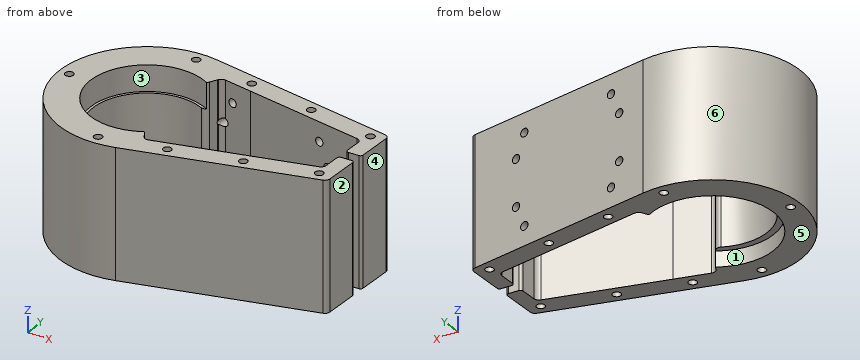
from build123d import *

# Parameters (mm, degrees)
EXTRUDE_1_DEPTH            = 50
SKETCH_2_R                 = 26
CUT_EXTRUDE_1_DEPTH        = 50
EXTRUDE_2_DEPTH            = 50
CUT_EXTRUDE_START          = -68
SKETCH_3_R                 = 1.6
CUT_EXTRUDE_2_DEPTH        = 68
CUT_EXTRUDE_1_2_DEPTH      = 143.467540163
CUT_EXTRUDE_1_2_DEPTH_BACK = 58
CUT_EXTRUDE_START_2        = -58
CUT_EXTRUDE_3_DEPTH        = 58
EXTRUDE_3_DEPTH            = 50
FILLET_1_R                 = 2
SKETCH_8_R                 = 22
CUT_EXTRUDE_4_DEPTH        = 10
SKETCH_9_R                 = 23.5
CUT_EXTRUDE_5_DEPTH        = 6
EXTRUDE_4_DEPTH            = 50
FILLET_2_R                 = 2
SKETCH_11_R                = 1.6
CUT_EXTRUDE_6_DEPTH        = 24
SKETCH_12_R                = 1.6
CUT_EXTRUDE_7_DEPTH        = 10
CUT_EXTRUDE_8_DEPTH        = 72
FILLET_3_R                 = 1


with BuildPart() as part:
    # 草图1 → 凸台-拉伸1 (new body)
    with BuildSketch(Plane.XY):
        with BuildLine():
            Line((-86.410526316, 32.89712665), (2.526315789, 9.675625485))
            ThreePointArc((2.526315789, 9.675625485), (10, 0), (2.526315789, -9.675625485))
            Line((2.526315789, -9.675625485), (-86.410526316, -32.89712665))
            ThreePointArc((-86.410526316, -32.89712665), (-129, 0), (-86.410526316, 32.89712665))
        make_face()
    extrude(amount=EXTRUDE_1_DEPTH)

    # 草图2 → Cut-Extrude 1 (cut)
    with BuildSketch(Plane.XY.offset(50)):
        with Locations((-95, 0)):
            Circle(SKETCH_2_R)
    extrude(amount=-CUT_EXTRUDE_1_DEPTH, mode=Mode.SUBTRACT)

    # 草图4 → 凸台-拉伸2 (add)
    with BuildSketch(Plane.XY.offset(50)):
        Polygon((-89.273684211, 33.514314964), (0, 18.260853628), (0, 0), align=None)
    extrude(amount=-EXTRUDE_2_DEPTH)

    # 草图3 → 切除-拉伸2 (cut)
    with BuildSketch(Plane.XY.offset(50).offset(CUT_EXTRUDE_START)):
        with Locations((-95, 30)):
            Circle(SKETCH_3_R)
        with Locations((-125, 0)):
            Circle(SKETCH_3_R)
        with Locations((-95, -30)):
            Circle(SKETCH_3_R)
        with Locations((-71.551753536, -24.883386101)):
            Circle(SKETCH_3_R)
        with Locations((-71.274432107, 26.380963088)):
            Circle(SKETCH_3_R)
        with Locations((-45.645838312, 22.002015719)):
            Circle(SKETCH_3_R)
        with Locations((-21.238501013, -11.746543996)):
            Circle(SKETCH_3_R)
        with Locations((-20.017244516, 17.623068351)):
            Circle(SKETCH_3_R)
        with Locations((-46.395127275, -18.314965049)):
            Circle(SKETCH_3_R)
        with BuildLine():
            Line((-67.233345602, -19.621745681), (-22.076558694, -7.831262064))
            Line((-22.076558694, -7.831262064), (-21.17859716, 13.763531668))
            Line((-21.17859716, 13.763531668), (-69.025115802, 21.938673408))
            ThreePointArc((-69.025115802, 21.938673408), (-61.031553592, 1.464461893), (-67.233345602, -19.621745681))
        make_face()
    extrude(amount=CUT_EXTRUDE_2_DEPTH, mode=Mode.SUBTRACT)

    # 草图5 → Cut-Extrude 1 2 (cut, two sides: drawn at the far end of the back side and taken through both)
    with BuildSketch(Plane.XY.offset(50).offset(-CUT_EXTRUDE_1_2_DEPTH_BACK)):
        Polygon((-16.353043274, -14.605045601), (-14.880678398, 20.803392951), (25.084784603, 19.141536445), (23.612419728, -16.266902106), align=None)
    extrude(amount=CUT_EXTRUDE_1_2_DEPTH + CUT_EXTRUDE_1_2_DEPTH_BACK, mode=Mode.SUBTRACT)

    # 草图6 → 切除-拉伸3 (cut)
    with BuildSketch(Plane.XY.offset(50).offset(CUT_EXTRUDE_START_2)):
        with BuildLine():
            Line((-90.621052632, 25.628593796), (-69.025115802, 21.938673408))
            ThreePointArc((-69.025115802, 21.938673408), (-61.031553592, 1.464461893), (-67.233345602, -19.621745681))
            Line((-67.233345602, -19.621745681), (-88.431578947, -25.156626262))
            ThreePointArc((-88.431578947, -25.156626262), (-69.024129218, 1.119882624), (-90.621052632, 25.628593796))
        make_face()
    extrude(amount=CUT_EXTRUDE_3_DEPTH, mode=Mode.SUBTRACT)

    # 草图7 → 凸台-拉伸3 (add)
    with BuildSketch(Plane.XY.offset(50)):
        with BuildLine():
            Line((-82, 22.516660498), (-84.5, 18.186533479))
            ThreePointArc((-84.5, 18.186533479), (-116, 0), (-84.5, -18.186533479))
            Line((-84.5, -18.186533479), (-82, -22.516660498))
            ThreePointArc((-82, -22.516660498), (-121, 0), (-82, 22.516660498))
        make_face()
    extrude(amount=-EXTRUDE_3_DEPTH)

    # 圆角1
    fillet_1_edges = [part.edges().sort_by_distance(p)[0] for p in [
        (-14.880678398, 20.803392951, 25),
        (-16.353043274, -14.605045601, 25),
        (-84.5, 18.186533479, 25),
        (-84.5, -18.186533479, 25),
        (-21.17859716, 13.763531668, 25),
        (-22.076558694, -7.831262064, 25),
    ]]
    fillet(fillet_1_edges, radius=FILLET_1_R)

    # 草图8 → 切除-拉伸4 (cut)
    with BuildSketch(Plane.XY.offset(50)):
        with Locations((-95, 0)):
            Circle(SKETCH_8_R)
    extrude(amount=-CUT_EXTRUDE_4_DEPTH, mode=Mode.SUBTRACT)

    # 草图9 → 切除-拉伸5 (cut)
    with BuildSketch(Plane(origin=(0, 0, 0), x_dir=(-1, 0, 0), z_dir=(0, 0, -1))):
        with Locations((95, 0)):
            Circle(SKETCH_9_R)
    extrude(amount=-CUT_EXTRUDE_5_DEPTH, mode=Mode.SUBTRACT)

    # 草图10 → 凸台-拉伸4 (add)
    with BuildSketch(Plane.XY.offset(50)):
        with BuildLine():
            Line((-90.621052632, 25.628593796), (-81.138728268, 24.008426897))
            Line((-81.138728268, 24.008426897), (-82, 22.516660498))
            ThreePointArc((-82, 22.516660498), (-86.172317115, 24.455510931), (-90.621052632, 25.628593796))
        make_face()
        with BuildLine():
            Line((-82, -22.516660498), (-81.518012702, -23.351486987))
            Line((-81.518012702, -23.351486987), (-88.431578947, -25.156626262))
            ThreePointArc((-88.431578947, -25.156626262), (-85.127151858, -24.052585507), (-82, -22.516660498))
        make_face()
    extrude(amount=-EXTRUDE_4_DEPTH)

    # 圆角2
    fillet_2_edges = [part.edges().sort_by_distance(p)[0] for p in [
        (-81.138728268, 24.008426897, 25),
        (-81.518012702, -23.351486987, 25),
    ]]
    fillet(fillet_2_edges, radius=FILLET_2_R)

    # 草图11 → 切除-拉伸6 (cut)
    with BuildSketch(Plane(origin=(3.031578947, 17.742872628, 0), x_dir=(0.9857151459881658, -0.16842105263157892, 0), z_dir=(0.16842105263157894, 0.9857151459881659, 0))):
        with Locations(Location((-37.931515403, -16, 0), (0, 0, 180))):
            Circle(SKETCH_11_R)
        with Locations(Location((-83.131515403, -16, 0), (0, 0, 180))):
            Circle(SKETCH_11_R)
        with Locations(Location((-83.131515403, -34, 0), (0, 0, 180))):
            Circle(SKETCH_11_R)
        with Locations(Location((-37.931515403, -34, 0), (0, 0, 180))):
            Circle(SKETCH_11_R)
    extrude(amount=-CUT_EXTRUDE_6_DEPTH, mode=Mode.SUBTRACT)

    # 草图12 → 切除-拉伸7 (cut)
    with BuildSketch(Plane(origin=(3.031578947, 17.742872628, 0), x_dir=(0.9857151459881658, -0.16842105263157892, 0), z_dir=(0.16842105263157894, 0.9857151459881659, 0))):
        with Locations(Location((-79.531515403, -7.5, 0), (0, 0, 180))):
            Circle(SKETCH_12_R)
        with Locations(Location((-41.531515403, -7.5, 0), (0, 0, 180))):
            Circle(SKETCH_12_R)
        with Locations(Location((-79.531515403, -42.5, 0), (0, 0, 180))):
            Circle(SKETCH_12_R)
        with Locations(Location((-41.531515403, -42.5, 0), (0, 0, 180))):
            Circle(SKETCH_12_R)
    extrude(amount=-CUT_EXTRUDE_7_DEPTH, mode=Mode.SUBTRACT)

    # 草图13 → 切除-拉伸8 (cut)
    with BuildSketch(Plane.XY.offset(50)):
        Polygon((-21.550135764, 4.82851696), (-15.539418673, 4.961555834), (-15.705941936, 0.956890399), (-21.716659027, 0.823851526), align=None)
    extrude(amount=-CUT_EXTRUDE_8_DEPTH, mode=Mode.SUBTRACT)

    # 圆角3
    fillet_3_edges = [part.edges().sort_by_distance(p)[0] for p in [
        (-15.705941936, 0.956890399, 25),
        (-15.539418673, 4.961555834, 25),
        (-21.716659027, 0.823851526, 25),
        (-21.550135764, 4.82851696, 25),
    ]]
    fillet(fillet_3_edges, radius=FILLET_3_R)


solid = part.part
Here's how the part is built. I have some questions about the finished solid (model axes, mm). Face numbers are marked on the shaded views. A direction names the side the tool comes from. Round coordinates to 2 decimals unless told otherwise and drop trailing zeros. Order: outer loops, then holes, each group sorted by start corner. A loop starts at its lowest first (then second) coordinate and runs counter-clockwise, first axis right, second up. Notation, with made-up numbers: (-5.5, 84) -> (48.5, 84) arc R15 cw to (48.5, 105) -> close; hole circle Ø5 at (69, 75). An arc over 180 degrees is marked (long way). Return JSON: item names as keys, results as strings.
Q1. If we section it at B-B on y = 8: List the corners of the cut face in (x, z) for me, plus the area to 3 significant figures.
Filled sheet:
{"outline": "(-128.05, 0) -> (-117.1, 0) -> (-117.1, 6) -> (-114.42, 6) -> (-114.42, 40) -> (-115.49, 40) -> (-115.49, 50) -> (-128.05, 50) -> close; (-21.42, 0) -> (-15.41, 0) -> (-15.41, 50) -> (-21.42, 50) -> close", "area": "955 mm^2"}
Q2. If we section it at C-C on x = -71.5: List the corners of the cut face in (y, z) for me.
Filled sheet:
{"outline": "(-29, 0) -> (-26.48, 0) -> (-26.48, 50) -> (-29, 50) -> close; (-23.28, 0) -> (-20.74, 0) -> (-20.74, 50) -> (-23.28, 50) -> close; (22.36, 0) -> (24.8, 0) -> (24.8, 50) -> (22.36, 50) -> close; (27.96, 0) -> (30.48, 0) -> (30.48, 50) -> (27.96, 50) -> close"}
Q3. For pin 1 Ø1.5 at (y, z) = (7, 5) entering from +X; pin 2 Ø5 at (x, y) = (-71.27, 26.38) entering from -Z; pin 3 Ø10 at (x, z) = (-98, 42.5) entering from -Y; pin 4 Ø5 at (x, z) = (-42, 25.5) entering from +Y, each with a flat end and sliding along its axis, tell me the tip position at first contact or that it passes through.
Filled sheet:
{"pin 1": "stops at x = -15.42", "pin 2": "stops at z = 0", "pin 3": "stops at y = -34", "pin 4": "stops at y = 25.86"}
Q4. If we section it at D-D on y = 30: Give the number of separate pieces and of enclosed holes in the cut face, plus the area to 3 significant figures.
Filled sheet:
{"separate pieces": "2", "enclosed holes": "4", "area": "1,920 mm^2"}
Q5. If we mould it in two halves opening along Y, with no side actions, what happens to the marked faces 3, 4, 5 and 6? For each: released by +Y, released by -Y, zero draft, split by the parting line, or undercut.
Filled sheet:
{"face 3": "undercut", "face 4": "released by -Y", "face 5": "zero draft", "face 6": "split by the parting line"}
Q6. I need wall thicknesses on line 1 along X through (y, z) = (0, 30); line 2 along X through (y, z) = (0, 44.5); line 3 along Y through (x, z) = (-95, 4). Which ranges of each line are inside material? Lowest first, please. Write a range as from..to.
Filled sheet:
{"line 1": "x = -129..-126.6, -123.4..-116, -21.74..-15.75", "line 2": "x = -129..-126.6, -123.4..-117, -21.74..-15.75", "line 3": "y = -34..-31.6, -28.4..-23.5, 23.5..28.4, 31.6..34"}
Q7. If we section it at A-A on x = -125: List the corners of the cut face in (y, z) for me, plus the area to 3 significant figures.
Filled sheet:
{"outline": "(-16, 0) -> (-1.6, 0) -> (-1.6, 50) -> (-16, 50) -> close; (1.6, 0) -> (16, 0) -> (16, 50) -> (1.6, 50) -> close", "area": "1,440 mm^2"}
Q8. Which directions (+Z, -Z, +X, -X, +Y, -Y) give clear straight access to the entire face, cutting with the end or side of a thin tool? Please do the marked faces 1 and 2.
Filled sheet:
{"face 1": "-Z", "face 2": "+Z, -Z, +X, -Y"}
